Autodesk Inventor part; units mm, degrees
ref_plane "YZ Plane" through (0, 0, 0) normal (1, 0, 0) x (0, 1, 0)
ref_plane "XZ Plane" through (0, 0, 0) normal (0, 1, 0) x (-1, 0, 0)
ref_plane "XY Plane" through (0, 0, 0) normal (0, 0, 1) x (1, 0, 0)
sketch "Sketch1" plane through (0, 0, 0) normal (0, 0, 1) x (1, 0, 0)
  line L0 (0, 0) -> (0, 65) construction
  circle A0 centre (0, 0) radius 11
  circle A1 centre (0, 65) radius 8.5
  line L1 (7.5, 17.4571) -> (-7.5, 17.4571)
  line L2 (-7.5, 17.4571) -> (-7.5, 53.1784)
  line L3 (-7.5, 53.1784) -> (7.5, 53.1784)
  line L4 (7.5, 53.1784) -> (7.5, 17.4571)
  line L5 (7.5, 17.4571) -> (-7.5, 53.1784) construction
  line L6 (-7.5, 17.4571) -> (7.5, 53.1784) construction
  arc A2 (7.5, 53.1784) -> (-7.5, 53.1784) centre (0, 65) ccw
  arc A3 (-7.5, 17.4571) -> (7.5, 17.4571) centre (0, 0) ccw
  point P0 (0, 35.3177)
  point P1 (0, 35.3177)
  dimension "d0" = 22
  dimension "d1" = 17
  dimension "d2" = 65
  dimension "d3" = 5.5
  dimension "d4" = 8
  dimension "d5" = 15
extrude "Extrusion1" add sketch "Sketch1" along normal blind 7
sketch "Sketch2" plane through (0, 0, 7) normal (0, 0, 1) x (1, 0, 0)
  circle A0 centre (0, 65) radius 8.5
  arc A1 (7.5, 53.1784) -> (-7.5, 53.1784) centre (0, 65) ccw
  circle A2 centre (0, 65) radius 14
extrude "Extrusion2" cut sketch "Sketch2" against normal blind 1
chamfer "Chamfer1" distance 1 angle 45 1 edges at (0, 51, 7)
properties part number "con rod"
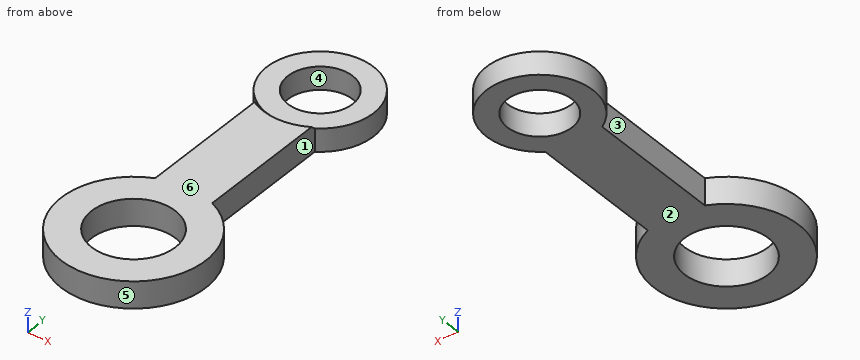
Could you check a few things on this model? Use its own coordinates, in mm. Face numbers are marked on the shaded views. A direction names the side the tool comes from. Coordinates: 2 decimals unless noted, no trailing zeros. Write each loop counter-clockwise with the first axis right and the second up, starting at its lowest first coordinate (ties: lowest second). Pieces come first, ordered by that corner, then holes. Notation, with made-up numbers: M 10,-35 L 19,-35 A20 cw 19,-20 Z; hole C 38,40 d8. An arc over 180 degrees is marked long. Answer as CSV lines item,"result". Start each with the question number.
1) I want a section at B-B, the plane z = 4.25. Please give me the cut outline in (x, y), and give its area (3 significant figures).
2) I want a section at C-C, the plane x = 0. Give the number of separate pieces and of enclosed holes in the cut face, and give its area (4 significant figures).
3) I want a section at A-A, the plane y = 65. Please give me the cut outline in (x, z), and give its area (3 significant figures).
4) Please list where these lines run through material, in increasing order: line 1 (Y direction, x = 0, z = 5.25); line 2 (Y direction, x = -1, z = 1.5); line 3 (Z direction, x = 9, y = 64). Write a range as from..to.
5) For the marked faces 1 and 2, which set-ups out of +Z, -Z, +X, -X, +Y, -Y let a thin tool reach every point of the face, with its end or its side?
6) I want a section at D-D, the plane y = 0. Please give me the cut outline in (x, z), and give its area (3 significant figures).
7) We'd pull the mould along X, two halves only. Please class the marked faces 3, 4, 5 and 6: +X half, -X half, draft (parallel to the pull), parting line (faces both ways), or undercut.
8) For P1, Ø2, axis at x = -9, z = 4, coming from the -Y side; P2, Ø4, axis at y = 68.5, z = 3.5, coming from the -X side, each with a flat end and sliding along its axis, tell me the tip position at first contact or that it passes through.
Data:
1,outline,"M -7.5,17.46 A19 ccw long 7.5,17.46 L 7.5,53.18 A14 ccw long -7.5,53.18 Z; hole C 0,0 d22; hole C 0,65 d17"
1,area,"1,640 mm^2"
2,separate pieces,"3"
2,enclosed holes,"0"
2,area,"401.5 mm^2"
3,outline,"M -14,0 L -8.5,0 L -8.5,6 L -14,6 Z; M 8.5,0 L 14,0 L 14,6 L 8.5,6 Z"
3,area,"66.0 mm^2"
4,line 1,"y = -19..-11, 11..56.5, 73.5..79"
4,line 2,"y = -18.97..-10.95, 10.95..56.56, 73.44..78.96"
4,line 3,"z = 0..6"
5,face 1,"+Z, -Z, +X"
5,face 2,"-Z, +X, -X, +Y, -Y"
6,outline,"M -19,0 L -11,0 L -11,7 L -19,7 Z; M 11,0 L 19,0 L 19,7 L 11,7 Z"
6,area,"112 mm^2"
7,face 3,"-X half"
7,face 4,"undercut"
7,face 5,"parting line"
7,face 6,"draft"
8,P1,"stops at y = -17.23"
8,P2,"stops at x = -13.92"
